from build123d import *

# Parameters (mm, degrees)
ESQUISSE1_W             = 130
ESQUISSE1_H             = 50
ESQUISSE1_R             = 2.1
ESQUISSE1_R_2           = 4.1
BOSS_EXTRU_1_DEPTH      = 3
ENL_V_MAT_EXTRU_1_REACH = 5
ESQUISSE2_W             = 30
ESQUISSE2_H             = 10


with BuildPart() as part:
    # Esquisse1 → Boss.-Extru.1 (new body)
    with BuildSketch(Plane.XY):
        with Locations((65, 25)):
            Rectangle(ESQUISSE1_W, ESQUISSE1_H)
        with Locations((4, 40)):
            Circle(ESQUISSE1_R, mode=Mode.SUBTRACT)
        with Locations((20, 40)):
            Circle(ESQUISSE1_R_2, mode=Mode.SUBTRACT)
        with Locations((36, 40)):
            Circle(ESQUISSE1_R, mode=Mode.SUBTRACT)
        with Locations((94, 40)):
            Circle(ESQUISSE1_R, mode=Mode.SUBTRACT)
        with Locations((110, 40)):
            Circle(ESQUISSE1_R_2, mode=Mode.SUBTRACT)
        with Locations((126, 40)):
            Circle(ESQUISSE1_R, mode=Mode.SUBTRACT)
        with Locations((5, 10)):
            Circle(ESQUISSE1_R, mode=Mode.SUBTRACT)
        with Locations((21, 10)):
            Circle(ESQUISSE1_R_2, mode=Mode.SUBTRACT)
        with Locations((37, 10)):
            Circle(ESQUISSE1_R, mode=Mode.SUBTRACT)
        with Locations((93, 10)):
            Circle(ESQUISSE1_R, mode=Mode.SUBTRACT)
        with Locations((109, 10)):
            Circle(ESQUISSE1_R_2, mode=Mode.SUBTRACT)
        with Locations((125, 10)):
            Circle(ESQUISSE1_R, mode=Mode.SUBTRACT)
        with BuildLine():
            Line((62.8, 10), (62.8, 40))
            ThreePointArc((62.8, 40), (65, 42.2), (67.2, 40))
            Line((67.2, 40), (67.2, 10))
            ThreePointArc((67.2, 10), (65, 7.8), (62.8, 10))
        make_face(mode=Mode.SUBTRACT)
    extrude(amount=BOSS_EXTRU_1_DEPTH)

    # Esquisse2 → Enlèv. mat.-Extru.1 (cut, up to next)
    with BuildSketch(Plane(origin=(0, 0, 0), x_dir=(-1, 0, 0), z_dir=(0, 0, -1)), mode=Mode.PRIVATE) as enl_v_mat_extru_1_sk1:
        with Locations((-15, 25)):
            Rectangle(ESQUISSE2_W, ESQUISSE2_H)
    enl_v_mat_extru_1_tool1 = extrude(enl_v_mat_extru_1_sk1.sketch, amount=-ENL_V_MAT_EXTRU_1_REACH, mode=Mode.PRIVATE) & part.part
    add(enl_v_mat_extru_1_tool1.solids().sort_by_distance((15, 25, 0))[0], mode=Mode.SUBTRACT)
    # Esquisse2 → Enlèv. mat.-Extru.1 (cut, up to next)
    with BuildSketch(Plane(origin=(0, 0, 0), x_dir=(-1, 0, 0), z_dir=(0, 0, -1)), mode=Mode.PRIVATE) as enl_v_mat_extru_1_sk2:
        with Locations((-115, 25)):
            Rectangle(ESQUISSE2_W, ESQUISSE2_H)
    enl_v_mat_extru_1_tool2 = extrude(enl_v_mat_extru_1_sk2.sketch, amount=-ENL_V_MAT_EXTRU_1_REACH, mode=Mode.PRIVATE) & part.part
    add(enl_v_mat_extru_1_tool2.solids().sort_by_distance((115, 25, 0))[0], mode=Mode.SUBTRACT)
    # Esquisse2 → Enlèv. mat.-Extru.1 (cut, up to next)
    with BuildSketch(Plane(origin=(0, 0, 0), x_dir=(-1, 0, 0), z_dir=(0, 0, -1)), mode=Mode.PRIVATE) as enl_v_mat_extru_1_sk3:
        with BuildLine():
            Line((-62.9, 50), (-67.1, 50))
            ThreePointArc((-67.1, 50), (-65, 47.9), (-62.9, 50))
        make_face()
    enl_v_mat_extru_1_tool3 = extrude(enl_v_mat_extru_1_sk3.sketch, amount=-ENL_V_MAT_EXTRU_1_REACH, mode=Mode.PRIVATE) & part.part
    add(enl_v_mat_extru_1_tool3.solids().sort_by_distance((65, 49.108732, 0))[0], mode=Mode.SUBTRACT)


solid = part.part
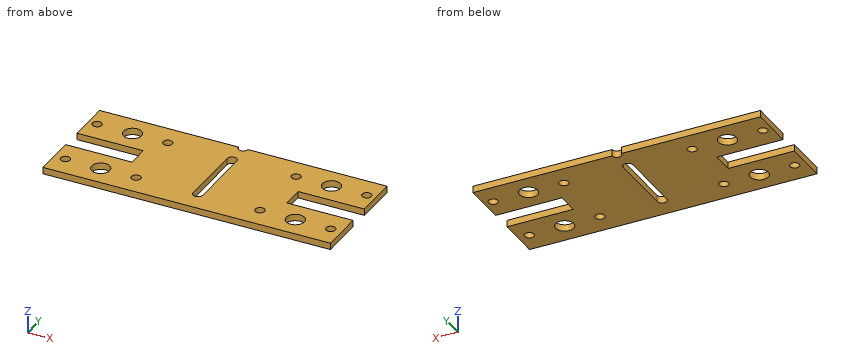
Can you work these out from the model? Positions are in its coordinate system, mm. Coordinates: 2 decimals unless noted, no trailing zeros. Order: outer loops, then holes, each group sorted by start corner. A loop starts at its lowest first (then second) coordinate and runs counter-clockwise, first axis right, second up. Notation, with made-up numbers: (61, 9) -> (68, 9) arc R19 ccw to (68, 21) -> close; hole circle Ø3 at (-20.75, 77.5). An arc over 180 degrees is marked (long way). Use one line per item in the form item = value.
Q1. Will these pins go through, and if not, where does the flat tip stop? P1, Ø3.5, axis at x = 93, y = 10, coming from the -Z side; P2, Ø6.5, axis at x = 94, y = 40, coming from the +Z side; P3, Ø1.5, axis at y = 23.5, z = 2.5, coming from the +X side.
From the geometry:
P1 = through
P2 = 3
P3 = 100
Q2. Imagine slicing it at C-C, the plane x = 36.5. List the corners of the cut face in (y, z) for me, then the cut area to 3 significant figures.
From the geometry:
outline = (0, 0) -> (7.96, 0) -> (7.96, 3) -> (0, 3) -> close; (12.04, 0) -> (37.96, 0) -> (37.96, 3) -> (12.04, 3) -> close; (42.04, 0) -> (50, 0) -> (50, 3) -> (42.04, 3) -> close
area = 126 mm²
Q3. Imagine slicing it at A-A, the plane z = 1.55. Give the number of separate pieces and of enclosed holes in the cut face, then the cut area to 3 significant figures.
From the geometry:
separate_pieces = 1
enclosed_holes = 13
area = 5,420 mm²
Q4. I need wall thicknesses on L1, parallel to Y at x = 20, z = 0.9; L2, parallel to X at y = 43.5, z = 0.6; L3, parallel to Y at x = 123.5, z = 0.55. Which ranges of each line are inside material? Lowest first, please.
From the geometry:
L1 = 0 to 6.02, 13.98 to 20, 30 to 35.9, 44.1 to 50
L2 = 0 to 17.86, 22.14 to 107.86, 112.14 to 130
L3 = 0 to 8.53, 11.47 to 20, 30 to 50
Q5. Imagine slicing it at B-B, the plane x = 20. List the corners of the cut face in (y, z) for me, then the cut area to 3 significant figures.
From the geometry:
outline = (0, 0) -> (6.02, 0) -> (6.02, 3) -> (0, 3) -> close; (13.98, 0) -> (20, 0) -> (20, 3) -> (13.98, 3) -> close; (30, 0) -> (35.9, 0) -> (35.9, 3) -> (30, 3) -> close; (44.1, 0) -> (50, 0) -> (50, 3) -> (44.1, 3) -> close
area = 71.5 mm²
